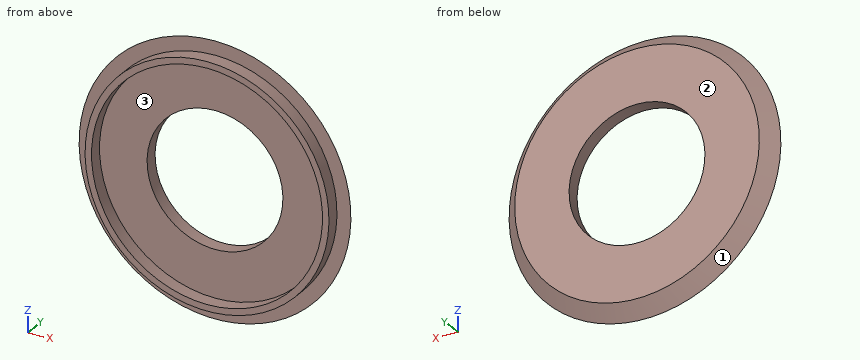
```python
from build123d import *

# Parameters (mm, degrees)
SKETCH1_R           = 100
BOSS_EXTRUDE1_DEPTH = 10
CHAMFER1_SIZE       = 10
SKETCH2_R           = 89.75
SKETCH2_R_2         = 85
BOSS_EXTRUDE2_DEPTH = 10
SKETCH3_R           = 50
CUT_EXTRUDE1_DEPTH  = 20


with BuildPart() as part:
    # Sketch1 → Boss-Extrude1 (new body)
    with BuildSketch(Plane(origin=(0, 0, 0), x_dir=(1, 0, 0), z_dir=(0, 1, 0))):
        with Locations(Location((0, 0, 0), (0, 0, 270))):
            Circle(SKETCH1_R)
    extrude(amount=BOSS_EXTRUDE1_DEPTH)

    # Chamfer1
    chamfer1_edges = [part.edges().sort_by_distance(p)[0] for p in [
        (0, 10, -100),
    ]]
    chamfer(chamfer1_edges, length=CHAMFER1_SIZE - 0.0001)  # a hair under: the kernel refuses the full size

    # Sketch2 → Boss-Extrude2 (add)
    with BuildSketch(Plane.XZ):
        with Locations(Location((0, 0, 0), (0, 0, 90))):
            Circle(SKETCH2_R)
        with Locations(Location((0, 0, 0), (0, 0, 270))):
            Circle(SKETCH2_R_2, mode=Mode.SUBTRACT)
    extrude(amount=BOSS_EXTRUDE2_DEPTH)

    # Sketch3 → Cut-Extrude1 (cut)
    with BuildSketch(Plane(origin=(0, 10, 0), x_dir=(1, 0, 0), z_dir=(0, 1, 0))):
        with Locations(Location((0, 0, 0), (0, 0, 270))):
            Circle(SKETCH3_R)
    extrude(amount=-CUT_EXTRUDE1_DEPTH, mode=Mode.SUBTRACT)


solid = part.part
```
CAD build for the part. Positions are in the model's coordinates, mm. Face numbers are marked on the shaded views. Give positions to 0.01 mm unless a question says otherwise; leave off trailing zeros. Order: outer loops, then holes, each group sorted by start corner. A loop starts at its lowest first (then second) coordinate and runs counter-clockwise, first axis right, second up.
(1) Drill centre lines: L1, parallel to X at y = -4.75, z = 0; L2, parallel to Y at x = 10.5, z = -61.5; L3, parallel to X at y = -7, z = 28. Where is each one in solid material? Low to high.
(2) Flat gauge pins, fed straight in: pin 1 (4 mm diameter, centred on y = -6, z = 53, fed in from -X); pin 2 (3 mm diameter, centred on y = -7, z = 61, fed in from -X); pin 3 (1.5 mm diameter, centred on y = -7.5, z = -25.5, fed in from +X). Where does each tip first touch, or does it go through?
(3) Mould opens along X. For the marked faces 1, 2 and 3 say: released by +X, released by -X, zero draft, split by the parting line, or undercut.
(4) Saw through at C-C, the plane y = -4. Give the cut face in (x, z), then the cut area to 3 significant figures.
Results found:
1. L1: x = -89.75 to -85, 85 to 89.75
1. L2: y = 0 to 10
1. L3: x = -85.27 to -80.26, 80.26 to 85.27
2. pin 1: stops at x = -73.85
2. pin 2: stops at x = -67.19
2. pin 3: stops at x = 86.27
3. face 1: split by the parting line
3. face 2: zero draft
3. face 3: undercut
4. outline: circle Ø179.5 at (0, 0); hole circle Ø170 at (0, 0)
4. area: 2,610 mm2
